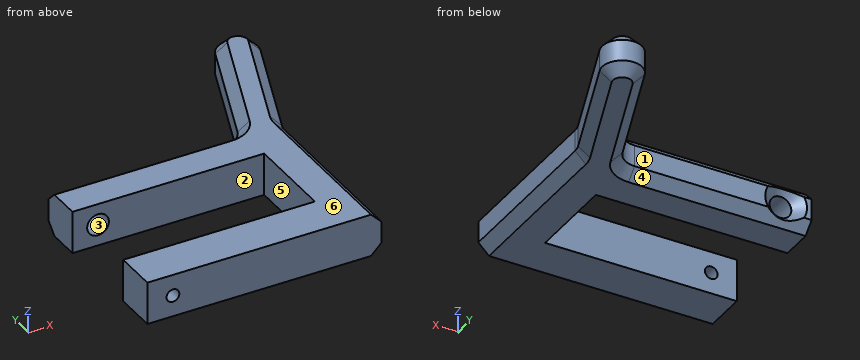
```python
from build123d import *

# Parameters (mm, degrees)
F1_DEPTH       = 10
F3_D           = 5.1
F3_DEPTH       = 20
F3_CSINK_D     = 9.8
F3_CSINK_ANGLE = 90
F3_TIP         = 1.5321945785
F5_D           = 3
F6_T1_DEPTH    = 29.0789805985
F6_T3_DEPTH    = 30.1186834219
F6_T5_DEPTH    = 47.9847156333
F6_T7_DEPTH    = 46.5081880684
F6_T10_ANGLE   = 180
F6_T12_ANGLE   = 180
F6_T14_ANGLE   = 69.1257858818
F6_T16_ANGLE   = 20.8742141182
F6_T18_ANGLE   = 69.1257858818
F6_T20_ANGLE   = 20.8742141182


# Not quite as in the source:
# - a fillet or chamfer that OpenCascade refuses, or shapes differently, is made with other operations: its cross-section is extruded or revolved along the edge and cut away or added


with BuildPart() as f1:
    # F0 (on Top) → F1 (new body)
    with BuildSketch(Plane.XY):
        with BuildLine():
            Line((41.5555081634, 20.5), (0, 20.5))
            Line((0, 20.5), (0, 10.5))
            Line((0, 10.5), (45, 10.5))
            Line((45, 10.5), (45, -10.5))
            Line((45, -10.5), (0, -10.5))
            Line((0, -10.5), (0, -20.5))
            Line((0, -20.5), (45, -20.5))
            Line((45, -20.5), (55, -20.5))
            Line((55, -20.5), (55, 19.5789805985))
            ThreePointArc((55, 19.5789805985), (55.0827282347, 20.4847611382), (55.3281753544, 21.3605682278))
            Line((55.3281753544, 21.3605682278), (65.6895257755, 48.5309478737))
            ThreePointArc((65.6895257755, 48.5309478737), (62.9889896705, 54.5607899764), (56.9591475677, 51.8602538715))
            Line((56.9591475677, 51.8602538715), (46.227332809, 23.7184123708))
            ThreePointArc((46.227332809, 23.7184123708), (44.3920608118, 21.382480228), (41.5555081634, 20.5))
        make_face()
    extrude(amount=F1_DEPTH)

    # F3
    with Locations(Plane(origin=(0, 20.5, 0), x_dir=(-1, 0, 0), z_dir=(0, 1, 0))):
        with Locations((-6, 5)):
            CounterSinkHole(F3_D / 2, F3_CSINK_D / 2, depth=F3_DEPTH, counter_sink_angle=F3_CSINK_ANGLE)
            with Locations((0, 0, -(F3_DEPTH + F3_TIP / 2))):  # 118° drill point
                Cone(0, F3_D / 2, F3_TIP, mode=Mode.SUBTRACT)

    # F5 (through all)
    with Locations(Plane(origin=(0, -10.5, 0), x_dir=(-1, 0, 0), z_dir=(0, 1, 0))):
        with Locations((-6, 5)):
            Hole(F5_D / 2)

    # F6: chamfer of 2.5 on 4 edges, made by hand

    # F6_s2 → F6_t1 (cut)
    with BuildSketch(Plane(origin=(14.1361725075, 37.0690265418, 0), x_dir=(0, 0, 1), z_dir=(0.3563175258, 0.9343649291, 0))):
        Polygon((10, 41.5855618218), (7.5, 44.0855618218), (10, 44.0855618218), align=None)
        Polygon((0, 41.5855618218), (2.5, 44.0855618218), (0, 44.0855618218), align=None)
    extrude(amount=F6_T1_DEPTH, mode=Mode.SUBTRACT)

    # F6_s4 → F6_t3 (cut)
    with BuildSketch(Plane(origin=(24.4975229285, 64.2394061877, 0), x_dir=(0, 0, 1), z_dir=(-0.3563175258, -0.9343649291, 0))):
        Polygon((7.5, -34.7419125306), (10, -37.2419125306), (10, -34.7419125306), align=None)
        Polygon((2.5, -34.7419125306), (0, -37.2419125306), (0, -34.7419125306), align=None)
    extrude(amount=F6_T3_DEPTH, mode=Mode.SUBTRACT)

    # F6_s6 → F6_t5 (cut)
    with BuildSketch(Plane.YZ.offset(-6.4292074699)):
        Polygon((20.5, 7.5), (18, 10), (20.5, 10), align=None)
        Polygon((20.5, 2.5), (18, 0), (20.5, 0), align=None)
    extrude(amount=F6_T5_DEPTH, mode=Mode.SUBTRACT)

    # F6_s8 → F6_t7 (cut)
    with BuildSketch(Plane.XZ.offset(-19.5789805985)):
        Polygon((52.5, 10), (55, 7.5), (55, 10), align=None)
        Polygon((52.5, 0), (55, 2.5), (55, 0), align=None)
    extrude(amount=F6_T7_DEPTH, mode=Mode.SUBTRACT)

    # F6_s9 → F6_t10 (revolve, cut)
    with BuildSketch(Plane(origin=(24.4975229285, 64.2394061877, 0), x_dir=(0, 0, 1), z_dir=(-0.3563175258, -0.9343649291, 0))):
        Polygon((0, -41.5855618218), (2.5, -44.0855618218), (0, -44.0855618218), align=None)
    revolve(axis=Axis((61.3243366716, 50.1956008726, 0), (0, 0, 1)), revolution_arc=F6_T10_ANGLE, mode=Mode.SUBTRACT)

    # F6_s11 → F6_t12 (revolve, cut)
    with BuildSketch(Plane(origin=(24.4975229285, 64.2394061877, 0), x_dir=(0, 0, 1), z_dir=(-0.3563175258, -0.9343649291, 0))):
        Polygon((10, -41.5855618218), (7.5, -44.0855618218), (10, -44.0855618218), align=None)
    revolve(axis=Axis((61.3243366716, 50.1956008726, 10), (0, 0, 1)), revolution_arc=F6_T12_ANGLE, mode=Mode.SUBTRACT)

    # F6_s13 → F6_t14 (revolve, cut)
    with BuildSketch(Plane(origin=(13.7657081698, 36.0975646869, 0), x_dir=(0, 0, 1), z_dir=(0.3563175258, 0.9343649291, 0))):
        Polygon((7.5, 34.7419125306), (10, 37.2419125306), (10, 34.7419125306), align=None)
    revolve(axis=Axis((41.5555081634, 25.5, 10), (0, 0, -1)), revolution_arc=F6_T14_ANGLE, mode=Mode.SUBTRACT)

    # F6_s15 → F6_t16 (revolve, cut)
    with BuildSketch(Plane.XZ.offset(-19.5789805985)):
        Polygon((52.5, 10), (55, 7.5), (55, 10), align=None)
    revolve(axis=Axis((60, 19.5789805985, 10), (0, 0, -1)), revolution_arc=F6_T16_ANGLE, mode=Mode.SUBTRACT)

    # F6_s17 → F6_t18 (revolve, cut)
    with BuildSketch(Plane(origin=(13.7657081698, 36.0975646869, 0), x_dir=(0, 0, 1), z_dir=(0.3563175258, 0.9343649291, 0))):
        Polygon((2.5, 34.7419125306), (0, 37.2419125306), (0, 34.7419125306), align=None)
    revolve(axis=Axis((41.5555081634, 25.5, 0), (0, 0, -1)), revolution_arc=F6_T18_ANGLE, mode=Mode.SUBTRACT)

    # F6_s19 → F6_t20 (revolve, cut)
    with BuildSketch(Plane.XZ.offset(-19.5789805985)):
        Polygon((52.5, 0), (55, 2.5), (55, 0), align=None)
    revolve(axis=Axis((60, 19.5789805985, 0), (0, 0, -1)), revolution_arc=F6_T20_ANGLE, mode=Mode.SUBTRACT)


solid = f1.part
```
Design review of the part built by this model. Coordinates are the model's own, in mm. Face numbers are marked on the shaded views. A direction names the side the tool comes from. Give positions to 0.01 mm unless a question says otherwise; leave off trailing zeros. Order: outer loops, then holes, each group sorted by start corner. A loop starts at its lowest first (then second) coordinate and runs counter-clockwise, first axis right, second up. Notation, with made-up numbers: (21, 52) -> (48, 52) arc R16 cw to (48, 71) -> close; hole circle Ø9 at (17, -19.75). An arc over 180 degrees is marked (long way). Write item = value, one per line. Start each with the question number.
(1) Mouldability with a two-part tool opening along Y and no side actions: class the marked faces 4, 5 and 6 as +Y half, -Y half, draft (parallel to the pull), parting line (faces both ways), or undercut.
(2) For the marked faces 1, 2 and 3, list the 3-axis set-ups (+Z, -Z, +X, -X, +Y, -Y) from which the entire face can be reached by the end or side of a thin tool; tool diameter is ignored.
(3) For pin 1 (4 mm diameter, centred on x = 6, z = 5, fed in from +Y); pin 2 (0.9 mm diameter, centred on x = 1, z = 5.5, fed in from +Y); pin 3 (6 mm diameter, centred on y = 46.5, z = 6.5, fed in from -X), all flat-tipped, find the tip position at first contact; note any pin that passes through.
(4) We need section A-A on z = 5. Write out the cut boundary in (x, y), plus the area to 3 significant figures.
(5) To check wall thickness, follow line 1 along Y through (x, z) = (37, 6.5); line 2 along Z through (x, y) = (6, 12.5); line 3 along Y through (x, z) = (35, 8.5). State the ranges of each line that lie inside material, in increasing order.
(6) We need section B-B on x = 6. Write out the cut boundary in (y, z).
(7) We need section C-C on y = 12. Write out the cut boundary in (x, z).
(8) We need section D-D on x = 31. Write out the cut boundary in (y, z).
Numbers:
q1.face_4 = +Y half
q1.face_5 = undercut
q1.face_6 = draft
q2.face_1 = +Z, -Z, -X, +Y
q2.face_2 = +Z, -Z, -X
q2.face_3 = +Y
q3.pin_1 = -10.5
q3.pin_2 = 20.5
q3.pin_3 = 53.77
q4.outline = (0, -20.5) -> (4.5, -20.5) -> (4.5, -10.5) -> (0, -10.5) -> close; (0, 10.5) -> (3.45, 10.5) -> (3.45, 18.15) -> (1.1, 20.5) -> (0, 20.5) -> close; (7.5, -20.5) -> (55, -20.5) -> (55, 19.58) arc R5 cw to (55.33, 21.36) -> (65.69, 48.53) arc R4.67 ccw to (56.96, 51.86) -> (46.23, 23.72) arc R5 cw to (41.56, 20.5) -> (10.9, 20.5) -> (8.55, 18.15) -> (8.55, 10.5) -> (45, 10.5) -> (45, -10.5) -> (7.5, -10.5) -> close
q4.area = 1,560 mm^2
q5.line_1 = -20.5 to -10.5, 10.5 to 20.5
q5.line_2 = 0 to 2.45, 7.55 to 10
q5.line_3 = -20.5 to -10.5, 10.5 to 19.5
q6.outline = (-20.5, 0) -> (-10.5, 0) -> (-10.5, 3.5) -> (-20.5, 3.5) -> close; (-20.5, 6.5) -> (-10.5, 6.5) -> (-10.5, 10) -> (-20.5, 10) -> close; (10.5, 0) -> (18, 0) -> (19.3, 1.3) -> (18.15, 2.45) -> (10.5, 2.45) -> close; (10.5, 7.55) -> (18.15, 7.55) -> (19.3, 8.7) -> (18, 10) -> (10.5, 10) -> close
q7.outline = (0, 0) -> (52.5, 0) -> (55, 2.5) -> (55, 7.5) -> (52.5, 10) -> (0, 10) -> close; hole circle Ø5.1 at (6, 5)
q8.outline = (-20.5, 0) -> (-10.5, 0) -> (-10.5, 10) -> (-20.5, 10) -> close; (10.5, 0) -> (18, 0) -> (20.5, 2.5) -> (20.5, 7.5) -> (18, 10) -> (10.5, 10) -> close
